Part model, mm, in its own coordinate system. Face numbers are marked on the shaded views. Round coordinates to 2 decimals unless told otherwise and drop trailing zeros. Write each loop counter-clockwise with the first axis right and the second up, starting at its lowest first coordinate (ties: lowest second). Pieces come first, ordered by that corner, then holes.
Autodesk Inventor part; units mm, degrees
ref_plane "Work Plane1" through (-10.6041, 0, 0) normal (0, -0.8660254, -0.5) x (1, 0, 0)
ref_plane "YZ Plane" through (0, 0, 0) normal (1, 0, 0) x (0, 1, 0)
ref_plane "XZ Plane" through (0, 0, 0) normal (0, 1, 0) x (-1, 0, 0)
sketch "Sketch1" plane through (0, 0, 0) normal (1, 0, 0) x (0, 1, 0)
  line L0 (-5.7735, 0) -> (-2.8868, 5)
  line L1 (-2.8868, 5) -> (2.8868, 5)
  line L2 (2.8868, 5) -> (5.7735, 0)
  line L3 (5.7735, 0) -> (2.8868, -5)
  line L4 (2.8868, -5) -> (-2.8868, -5)
  line L5 (-2.8868, -5) -> (-5.7735, 0)
  point P0 (0, 0)
  point P1 (0, 0)
  dimension "d0" = 11.547
extrude "Body" add sketch "Sketch1" along normal blind 5.7
sketch "Sketch2" plane through (0, 0, 0) normal (0, 0, 1) x (1, 0, 0)
  line L0 (0, 2.8868) -> (0, 5.7735)
  line L1 (0, 5.7735) -> (5.7, 5.7735)
  line L2 (5.7, 2.8868) -> (5.7, 5.7735)
  line L3 (-1.14, 0) -> (6.84, 0)
  line L4 (0.4466, 5.7735) -> (0, 5)
  line L5 (5.2534, 5.7735) -> (5.7, 5)
  dimension "d3" = 30
  dimension "d4" = 30
  dimension "d5" = 10
  dimension "d6" = 10
revolve "Chamfer1" cut sketch "Sketch2" angle 360 about axis through (-10, 0, 0) along (1, 0, 0)
sketch "Sketch3" plane through (5.7, 0, 0) normal (1, 0, 0) x (0, 0, -1)
  arc A0 (-2.5, -4.3301) -> (2.5, -4.3301) centre (0, 0) ccw
hole "Thread" at (5.7, 0, 0) direction (-1, 0, 0) diameter 4.917 end through all
chamfer "Chamfer2" distance 0.5413 angle 30 1 edges at (5.7, 0, 2.4585) measured on face at (5.7, -4.1286, -0.0988)
chamfer "Chamfer3" distance 0.5413 angle 30 1 edges at (0, 0, 2.4585) measured on face at (0, -4.1286, -0.0988)
ref_plane "Work Plane1" through (-10.6041, 0, 0) normal (0, -0.8660254, -0.5) x (1, 0, 0)
equation "\"d0\" = 1.1547 * SW"
equation "\"d1\" = KOH"
equation "\"d3\" = ANG1"
equation "\"d4\" = ANG2"
equation "\"d5\" = SW0"
equation "\"d6\" = SW01"
equation "\"d8\" = -0.5 * GD1 + 0.5 * NND"
equation "\"d40\" = -0.5 * GD1 + 0.5 * NND"
equation "\"d10\" = -0.5 * GD1 + 0.5 * NND"
equation "\"d41\" = -0.5 * GD1 + 0.5 * NND"
equation "\"ANG1\" = 30deg"
equation "\"ANG2\" = 30deg"
equation "\"NND\" = 6"
equation "\"KOH\" = 5.7"
equation "\"SW0\" = SW"
equation "\"SW01\" = SW"
equation "\"GUL\" = 0.541266 * PTC"
equation "\"THREADDIA\" = 6"
equation "\"TOA\" = 30deg"
equation "\"PTC\" = 1"
equation "\"E0\" = 1.155 * SW"
equation "\"GAL\" = 0.541266 * PTC"
properties part number "Nut GB/T 6175 M6" material "Steel, Mild"
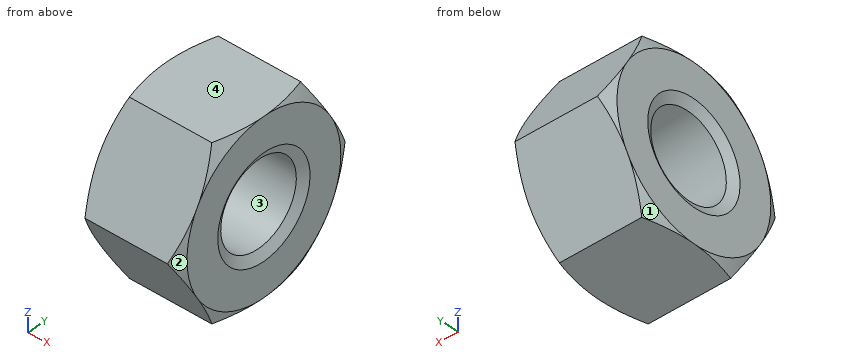
Q1. Wall check: L1, parallel to Z at x = 1.4, y = 0; L2, parallel to Y at x = 3.7, z = -0.75; L3, parallel to Z at x = 2.1, y = -1.5. Give the ranges that are in metal, low to high.
Values follow:
L1: z = -5 to -2.46, 2.46 to 5
L2: y = -5.34 to -2.34, 2.34 to 5.34
L3: z = -5 to -1.95, 1.95 to 5
Q2. Mould opens along Y. For the marked faces 1, 2, 3 and 4 say: +Y half, -Y half, draft (parallel to the pull), parting line (faces both ways), or undercut.
Values follow:
face 1: +Y half
face 2: -Y half
face 3: undercut
face 4: draft
Q3. Drop flat-ended pins along their axis: pin 1 (1.5 mm diameter, centred on x = 3, z = -2, fed in from -Y); pin 2 (2 mm diameter, centred on x = 1.5, z = -2.5, fed in from +Y); pin 3 (1.5 mm diameter, centred on x = 2, z = -2.5, fed in from -Y); pin 4 (3 mm diameter, centred on y = 0, z = 0, fed in from +X). Give the stop position or say it passes through.
Values follow:
pin 1: stops at y = -5.05
pin 2: stops at y = 4.91
pin 3: stops at y = -4.76
pin 4: passes through
Q4. Cut at A-A on x = 1.95. Write the cut outline in (y, z), plus the area to 3 significant figures.
Values follow:
outline: (-5.77, 0) - (-2.89, -5) - (2.89, -5) - (5.77, 0) - (2.89, 5) - (-2.89, 5) - close; hole circle Ø4.92 at (0, 0)
area: 67.6 mm2
